Model file for the job. Use its own axes, mm. A direction names the side the tool comes from. Round coordinates to 2 decimals unless told otherwise and drop trailing zeros. Put each result on its own line as item: value. Start each with the question number.
Q1. Pull direction Y, two halves, no side cores. Call faces 4 (the face through (11.78, 3.71, -0.44)), 5 (the face through (0.015, 10.785, 0.138)), 6 (the face through (-0.08, -6.42, 0.6)), 7 (the face through (-0.1, -12.5, 0)): released by +Y, released by -Y, zero draft, split by the parting line, or undercut.
Q2. Probe L1, parallel to Y at x = 8, z = -0.2; L2, parallel to Y at x = -8, z = -1.4; L3, parallel to X at y = -10.5, z = 0.95. List the from-to ranges inside material, lowest first.
Q3. 3-axis set-ups, long thin cutter, end or side, ignore diameter. For faces 1 (the face through (4.25, 0, -1)), 2 (the face through (4.65, -0.1, 0.58)), 3 (the face through (5, 0, -1.5)): which of +Z, -Z, +X, -X, +Y, -Y reach the whole face in a straight line?
Q4. Flat gauge pins, fed straight in: P1, Ø0.7, axis at x = 1, z = -0.5, coming from the +Y side; P2, Ø1, axis at x = 4.5, z = 0.5, coming from the +Y side; P3, Ø2, axis at x = 1.5, y = -6, coming from the +Z side. Where does each tip first touch, or does it go through?
from build123d import *
from OCP.BRepFilletAPI import BRepFilletAPI_MakeChamfer

# Parameters (mm, degrees)
SKETCH1_R           = 12.35
SKETCH1_R_2         = 1.7
BOSS_EXTRUDE1_DEPTH = 1.5
BOSS_EXTRUDE3_START = 1
SKETCH3_R           = 13.5
SKETCH3_R_2         = 1.7
BOSS_EXTRUDE3_DEPTH = 1
CHAMFER2_SIZE       = 0.5
CHAMFER3_SIZE       = 2
CHAMFER3_SIZE2      = 1.400415076
SKETCH2_W           = 8.5
SKETCH2_H           = 12
CUT_EXTRUDE2_DEPTH  = 20.254869514
CHAMFER4_SIZE       = 0.2
CHAMFER5_SIZE       = 0.6
FILLET1_START       = -6
FILLET1_DEPTH       = 12
FILLET1_START_2     = -5.6500001
FILLET1_2_DEPTH     = 11.3000001
FILLET1_START_3     = -8
FILLET1_3_DEPTH     = 2
FILLET1_START_4     = 6
FILLET1_4_DEPTH     = 2
CUT_EXTRUDE3_DEPTH  = 1
FILLET2_R           = 1


with BuildPart() as part:
    # Sketch1 → Boss-Extrude1 (new body)
    with BuildSketch(Plane.XY):
        Circle(SKETCH1_R)
        with Locations((-8, 0)):
            Circle(SKETCH1_R_2, mode=Mode.SUBTRACT)
        with Locations(Location((8, 0, 0), (0, 0, 180))):
            Circle(SKETCH1_R_2, mode=Mode.SUBTRACT)
    extrude(amount=-BOSS_EXTRUDE1_DEPTH)

    # Sketch3 → Boss-Extrude3 (add)
    with BuildSketch(Plane.XY.offset(BOSS_EXTRUDE3_START)):
        Circle(SKETCH3_R)
        with Locations((-8, 0)):
            Circle(SKETCH3_R_2, mode=Mode.SUBTRACT)
        with Locations((8, 0)):
            Circle(SKETCH3_R_2, mode=Mode.SUBTRACT)
    extrude(amount=-BOSS_EXTRUDE3_DEPTH)

    # Chamfer2
    chamfer2_edges = [part.edges().sort_by_distance(p)[0] for p in [
        (-13.5, 0, 0),
    ]]
    chamfer(chamfer2_edges, length=CHAMFER2_SIZE)

    # Chamfer3: one chamfer whose edges measure the first distance from different faces: ONE call of the kernel's chamfer builder (chamfer() names one face for all edges)
    chamfer3_edges_1 = [part.edges().sort_by_distance(p)[0] for p in [
        (-9.7, 0, 1),
    ]]
    chamfer3_side_1 = [part.faces().sort_by_distance(p)[0] for p in [
        (-9.7, 0, -0.25),
    ]]
    chamfer3_edges_2 = [part.edges().sort_by_distance(p)[0] for p in [
        (6.3, 0, 1),
    ]]
    chamfer3_side_2 = [part.faces().sort_by_distance(p)[0] for p in [
        (8, -1.7, -0.25),
    ]]
    chamfer3 = BRepFilletAPI_MakeChamfer(part.part.solid().wrapped)
    for e in chamfer3_edges_1:
        chamfer3.Add(CHAMFER3_SIZE, CHAMFER3_SIZE2, e.wrapped, chamfer3_side_1[0].wrapped)  # the first distance lies on this face
    for e in chamfer3_edges_2:
        chamfer3.Add(CHAMFER3_SIZE, CHAMFER3_SIZE2, e.wrapped, chamfer3_side_2[0].wrapped)  # the first distance lies on this face
    add(Compound.cast(chamfer3.Shape()), mode=Mode.REPLACE)

    # Sketch2 → Cut-Extrude2 (cut, through all)
    with BuildSketch(Plane(origin=(0, 0, -1.5), x_dir=(-1, 0, 0), z_dir=(0, 0, -1))):
        Rectangle(SKETCH2_W, SKETCH2_H)
    extrude(amount=-CUT_EXTRUDE2_DEPTH, mode=Mode.SUBTRACT)

    # Chamfer4
    chamfer4_edges = [part.edges().sort_by_distance(p)[0] for p in [
        (-4.25, 0, -1.5),
        (0, 6, -1.5),
        (4.25, 0, -1.5),
        (0, -6, -1.5),
    ]]
    chamfer(chamfer4_edges, length=CHAMFER4_SIZE)

    # Chamfer5
    chamfer5_edges = [part.edges().sort_by_distance(p)[0] for p in [
        (-12.35, 0, -1.5),
    ]]
    chamfer(chamfer5_edges, length=CHAMFER5_SIZE)

    # Fillet1: read off the stored shape, not the designer's step
    # Fillet1 outline → Fillet1 (cut)
    with BuildSketch(Plane(origin=(0, 0, 0), x_dir=(1, 0, 0), z_dir=(0, 1, 0)).offset(FILLET1_START)):
        with BuildLine():
            Line((-5.65, -1), (-4.25, -1))
            Line((-4.25, -1), (-4.25, 0.4))
            ThreePointArc((-4.25, 0.4), (-4.660050506, -0.589949494), (-5.65, -1))
        make_face()
        with BuildLine():
            ThreePointArc((5.65, -1), (4.660050506, -0.589949494), (4.25, 0.4))
            Line((4.25, 0.4), (4.25, -1))
            Line((4.25, -1), (5.65, -1))
        make_face()
    extrude(amount=FILLET1_DEPTH, mode=Mode.SUBTRACT)

    # Fillet1 2 outline → Fillet1 2 (cut)
    with BuildSketch(Plane.YZ.offset(FILLET1_START_2)):
        with BuildLine():
            Line((7.4, 1), (6, 1))
            Line((6, 1), (6, -0.4))
            ThreePointArc((6, -0.4), (6.410050506, 0.589949494), (7.4, 1))
        make_face()
        with BuildLine():
            ThreePointArc((-7.4, 1), (-6.410050506, 0.589949494), (-6, -0.4))
            Line((-6, -0.4), (-6, 1))
            Line((-6, 1), (-7.4, 1))
        make_face()
    extrude(amount=FILLET1_2_DEPTH, mode=Mode.SUBTRACT)

    # Fillet1 3 outline → Fillet1 3 (add)
    with BuildSketch(Plane(origin=(0, 0, 0), x_dir=(1, 0, 0), z_dir=(0, 1, 0)).offset(FILLET1_START_3)):
        with BuildLine():
            ThreePointArc((4.25, 0.4), (4.660050506, -0.589949494), (5.65, -1))
            Line((5.65, -1), (5.65, 0.4))
            Line((5.65, 0.4), (4.25, 0.4))
        make_face()
        with BuildLine():
            Line((-5.6500001, 0.4), (-5.65, -1))
            ThreePointArc((-5.65, -1), (-4.660050506, -0.589949494), (-4.25, 0.4))
            Line((-4.25, 0.4), (-5.6500001, 0.4))
        make_face()
    extrude(amount=FILLET1_3_DEPTH)

    # Fillet1 4 outline → Fillet1 4 (add)
    with BuildSketch(Plane(origin=(0, 0, 0), x_dir=(1, 0, 0), z_dir=(0, 1, 0)).offset(FILLET1_START_4)):
        with BuildLine():
            ThreePointArc((4.25, 0.4), (4.660050506, -0.589949494), (5.65, -1))
            Line((5.65, -1), (5.65, 0.4))
            Line((5.65, 0.4), (4.25, 0.4))
        make_face()
        with BuildLine():
            Line((-5.6500001, 0.4), (-5.65, -1))
            ThreePointArc((-5.65, -1), (-4.660050506, -0.589949494), (-4.25, 0.4))
            Line((-4.25, 0.4), (-5.6500001, 0.4))
        make_face()
    extrude(amount=FILLET1_4_DEPTH)

    # Sketch4 → Cut-Extrude3 (cut)
    with BuildSketch(Plane.XY.offset(1)):
        with BuildLine():
            Line((-1.07681329, 11.278202352), (1.07681329, 11.278202352))
            ThreePointArc((1.07681329, 11.278202352), (2.210300963, 10.144714678), (1.07681329, 9.011227005))
            Line((1.07681329, 9.011227005), (-1.07681329, 9.011227005))
            ThreePointArc((-1.07681329, 9.011227005), (-2.210300963, 10.144714678), (-1.07681329, 11.278202352))
        make_face()
        with BuildLine():
            Line((-1.07681329, -11.278202352), (1.07681329, -11.278202352))
            ThreePointArc((1.07681329, -11.278202352), (2.210300963, -10.144714678), (1.07681329, -9.011227005))
            Line((1.07681329, -9.011227005), (-1.07681329, -9.011227005))
            ThreePointArc((-1.07681329, -9.011227005), (-2.210300963, -10.144714678), (-1.07681329, -11.278202352))
        make_face()
    extrude(amount=-CUT_EXTRUDE3_DEPTH, mode=Mode.SUBTRACT)

    # Fillet2
    fillet2_edges = [part.edges().sort_by_distance(p)[0] for p in [
        (2.210300963, -10.144714678, 0),
        (0, -11.278202352, 0),
        (-2.210300963, -10.144714678, 0),
        (0, -9.011227005, 0),
        (2.210300963, 10.144714678, 0),
        (0, 9.011227005, 0),
        (-2.210300963, 10.144714678, 0),
        (0, 11.278202352, 0),
    ]]
    fillet(fillet2_edges, radius=FILLET2_R - 0.0001)  # a hair under: the kernel refuses the full size

    # Chamfer6: read off the stored shape, not the designer's step
    # Chamfer6: loft between two sections, ruled curve by curve
    chamfer6_from = [
        Edge.make_three_point_arc((-1.07681329, 11.144227755, 0.5), (-1.783575765, 10.851477153, 0.5), (-2.076326367, 10.144714678, 0.5)),
        Edge.make_three_point_arc((-2.076326367, 10.144714678, 0.5), (-1.783575765, 9.437952203, 0.5), (-1.07681329, 9.145201601, 0.5)),
        Edge.make_three_point_arc((1.07681329, 9.145201601, 0.5), (1.783575765, 9.437952203, 0.5), (2.076326367, 10.144714678, 0.5)),
        Edge.make_three_point_arc((2.076326367, 10.144714678, 0.5), (1.783575765, 10.851477153, 0.5), (1.07681329, 11.144227755, 0.5)),
        Edge.make_line((1.07681329, 11.144227755, 0.5), (-1.07681329, 11.144227755, 0.5)),
        Edge.make_line((-1.07681329, 9.145201601, 0.5), (1.07681329, 9.145201601, 0.5)),
    ]
    chamfer6_to = [
        Edge.make_three_point_arc((-1.07681329, 12.010253159, 1), (-2.3959482, 11.463849589, 1), (-2.942351771, 10.144714678, 1)),
        Edge.make_three_point_arc((-2.942351771, 10.144714678, 1), (-2.3959482, 8.825579768, 1), (-1.07681329, 8.279176197, 1)),
        Edge.make_three_point_arc((1.07681329, 8.279176197, 1), (2.3959482, 8.825579768, 1), (2.942351771, 10.144714678, 1)),
        Edge.make_three_point_arc((2.942351771, 10.144714678, 1), (2.3959482, 11.463849589, 1), (1.07681329, 12.010253159, 1)),
        Edge.make_line((1.07681329, 12.010253159, 1), (-1.07681329, 12.010253159, 1)),
        Edge.make_line((-1.07681329, 8.279176197, 1), (1.07681329, 8.279176197, 1)),
    ]
    chamfer6 = Solid(Shell([*[Face.make_surface_from_curves(chamfer6_from[k], chamfer6_to[k]) for k in range(6)], Face(Wire(chamfer6_from)), Face(Wire(chamfer6_to))]))
    add(chamfer6, mode=Mode.SUBTRACT)

    # Chamfer6 2: loft between two sections, ruled curve by curve
    chamfer6_2_from = [
        Edge.make_three_point_arc((-1.07681329, -9.145201601, 0.5), (-1.783575765, -9.437952203, 0.5), (-2.076326367, -10.144714678, 0.5)),
        Edge.make_three_point_arc((-2.076326367, -10.144714678, 0.5), (-1.783575765, -10.851477153, 0.5), (-1.07681329, -11.144227755, 0.5)),
        Edge.make_three_point_arc((1.07681329, -11.144227755, 0.5), (1.783575765, -10.851477153, 0.5), (2.076326367, -10.144714678, 0.5)),
        Edge.make_three_point_arc((2.076326367, -10.144714678, 0.5), (1.783575765, -9.437952203, 0.5), (1.07681329, -9.145201601, 0.5)),
        Edge.make_line((1.07681329, -9.145201601, 0.5), (-1.07681329, -9.145201601, 0.5)),
        Edge.make_line((-1.07681329, -11.144227755, 0.5), (1.07681329, -11.144227755, 0.5)),
    ]
    chamfer6_2_to = [
        Edge.make_three_point_arc((-1.07681329, -8.279176197, 1), (-2.3959482, -8.825579768, 1), (-2.942351771, -10.144714678, 1)),
        Edge.make_three_point_arc((-2.942351771, -10.144714678, 1), (-2.3959482, -11.463849589, 1), (-1.07681329, -12.010253159, 1)),
        Edge.make_three_point_arc((1.07681329, -12.010253159, 1), (2.3959482, -11.463849589, 1), (2.942351771, -10.144714678, 1)),
        Edge.make_three_point_arc((2.942351771, -10.144714678, 1), (2.3959482, -8.825579768, 1), (1.07681329, -8.279176197, 1)),
        Edge.make_line((1.07681329, -8.279176197, 1), (-1.07681329, -8.279176197, 1)),
        Edge.make_line((-1.07681329, -12.010253159, 1), (1.07681329, -12.010253159, 1)),
    ]
    chamfer6_2 = Solid(Shell([*[Face.make_surface_from_curves(chamfer6_2_from[k], chamfer6_2_to[k]) for k in range(6)], Face(Wire(chamfer6_2_from)), Face(Wire(chamfer6_2_to))]))
    add(chamfer6_2, mode=Mode.SUBTRACT)


solid = part.part
Ans:
1. face 4: split by the parting line
1. face 5: undercut
1. face 6: undercut
1. face 7: zero draft
2. L1: y = -9.41 to -2.26, 2.26 to 9.41
2. L2: y = -8.74 to -1.7, 1.7 to 8.74
2. L3: x = -8.49 to -2.82, 2.82 to 8.49
3. face 1: +Z, -Z
3. face 2: +Z
3. face 3: -Z, +X, -X, +Y, -Y
4. P1: stops at y = 12.33
4. P2: stops at y = 12.89
4. P3: stops at z = 0.94
